Design review of the part built by this model. Coordinates are the model's own, in mm. Coordinates: 2 decimals unless noted, no trailing zeros. Order: outer loops, then holes, each group sorted by start corner. A loop starts at its lowest first (then second) coordinate and runs counter-clockwise, first axis right, second up.
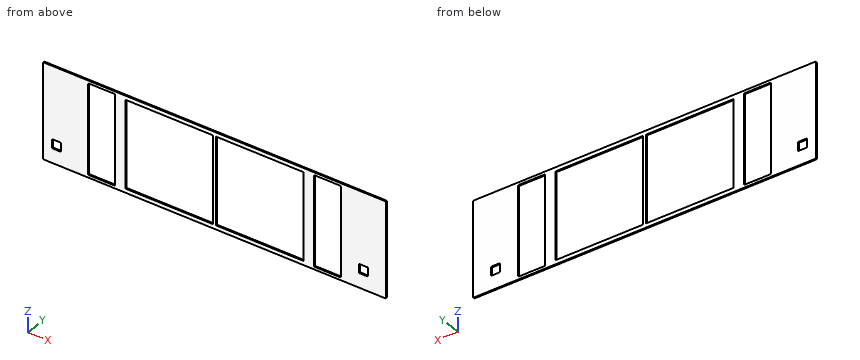
from build123d import *

# Parameters (mm, degrees)
SKETCH_1_W      = 194
SKETCH_1_H      = 194
EXTRUDE_1_DEPTH = 3


with BuildPart() as part:
    # 草图1 → 凸台-拉伸1 (new body)
    with BuildSketch(Plane(origin=(0, 0, 0), x_dir=(1, 0, 0), z_dir=(0, 1, 0))):
        with BuildLine():
            Line((2, 0), (758, 0))
            ThreePointArc((758, 0), (759.414213562, 0.585786438), (760, 2))
            Line((760, 2), (760, 210))
            ThreePointArc((760, 210), (759.414213562, 211.414213562), (758, 212))
            Line((758, 212), (2, 212))
            ThreePointArc((2, 212), (0.585786438, 211.414213562), (0, 210))
            Line((0, 210), (0, 2))
            ThreePointArc((0, 2), (0.585786438, 0.585786438), (2, 0))
        make_face()
        with Locations((480, 106)):
            Rectangle(SKETCH_1_W, SKETCH_1_H, mode=Mode.SUBTRACT)
        with Locations((280, 106)):
            Rectangle(SKETCH_1_W, SKETCH_1_H, mode=Mode.SUBTRACT)
        with BuildLine():
            Line((658, 6), (602, 6))
            ThreePointArc((602, 6), (600.585786438, 6.585786438), (600, 8))
            Line((600, 8), (600, 204))
            ThreePointArc((600, 204), (600.585786438, 205.414213562), (602, 206))
            Line((602, 206), (658, 206))
            ThreePointArc((658, 206), (659.414213562, 205.414213562), (660, 204))
            Line((660, 204), (660, 8))
            ThreePointArc((660, 8), (659.414213562, 6.585786438), (658, 6))
        make_face(mode=Mode.SUBTRACT)
        with BuildLine():
            Line((158, 6), (102, 6))
            ThreePointArc((102, 6), (100.585786438, 6.585786438), (100, 8))
            Line((100, 8), (100, 204))
            ThreePointArc((100, 204), (100.585786438, 205.414213562), (102, 206))
            Line((102, 206), (158, 206))
            ThreePointArc((158, 206), (159.414213562, 205.414213562), (160, 204))
            Line((160, 204), (160, 8))
            ThreePointArc((160, 8), (159.414213562, 6.585786438), (158, 6))
        make_face(mode=Mode.SUBTRACT)
        with BuildLine():
            Line((718, 160), (702, 160))
            ThreePointArc((702, 160), (700.585786438, 160.585786438), (700, 162))
            Line((700, 162), (700, 178))
            ThreePointArc((700, 178), (700.585786438, 179.414213562), (702, 180))
            Line((702, 180), (718, 180))
            ThreePointArc((718, 180), (719.414213562, 179.414213562), (720, 178))
            Line((720, 178), (720, 162))
            ThreePointArc((720, 162), (719.414213562, 160.585786438), (718, 160))
        make_face(mode=Mode.SUBTRACT)
        with BuildLine():
            Line((38, 160), (22, 160))
            ThreePointArc((22, 160), (20.585786438, 160.585786438), (20, 162))
            Line((20, 162), (20, 178))
            ThreePointArc((20, 178), (20.585786438, 179.414213562), (22, 180))
            Line((22, 180), (38, 180))
            ThreePointArc((38, 180), (39.414213562, 179.414213562), (40, 178))
            Line((40, 178), (40, 162))
            ThreePointArc((40, 162), (39.414213562, 160.585786438), (38, 160))
        make_face(mode=Mode.SUBTRACT)
    extrude(amount=-EXTRUDE_1_DEPTH)


solid = part.part
1. Add section D-D (y = -2.25). State how many separate pieces and enclosed holes the cut face has, and give its area (3 significant figures).
2. Add section B-B (z = -49). Give the boundary of the cut face in (x, y).
3. Add section C-C (x = 145). Give the boundary of the cut face in (y, z), and give its area (3 significant figures).
4. Add section A-A (x = 496.5). Give the boundary of the cut face in (y, z).
5. To check wall thickness, follow line 1 (X direction, y = -0.95, z = -56.5); line 2 (Z direction, x = 292, y = -2.8); line 3 (Z direction, x = 113, y = -0.4). State the ranges of each line that lie inside material, in increasing order.
Solution:
1. separate pieces: 1
1. enclosed holes: 6
1. area: 61,100 mm2
2. outline: (0, -3) - (100, -3) - (100, 0) - (0, 0) - close; (160, -3) - (183, -3) - (183, 0) - (160, 0) - close; (377, -3) - (383, -3) - (383, 0) - (377, 0) - close; (577, -3) - (600, -3) - (600, 0) - (577, 0) - close; (660, -3) - (760, -3) - (760, 0) - (660, 0) - close
3. outline: (-3, -212) - (0, -212) - (0, -206) - (-3, -206) - close; (-3, -6) - (0, -6) - (0, 0) - (-3, 0) - close
3. area: 36.0 mm2
4. outline: (-3, -212) - (0, -212) - (0, -203) - (-3, -203) - close; (-3, -9) - (0, -9) - (0, 0) - (-3, 0) - close
5. line 1: x = 0 to 100, 160 to 183, 377 to 383, 577 to 600, 660 to 760
5. line 2: z = -212 to -203, -9 to 0
5. line 3: z = -212 to -206, -6 to 0
